Design review of the part built by this model. Coordinates are the model's own, in mm. Face numbers are marked on the shaded views. A direction names the side the tool comes from. Round coordinates to 2 decimals unless told otherwise and drop trailing zeros. Loops run counter-clockwise (first coordinate to the right, second up) from the corner with the lowest first, then second, coordinate; pieces in that order, holes last. Notation, with made-up numbers: (-17.75, 54) - (14.25, 54) arc R20 ccw to (14.25, 84) - close; hole circle Ø10 at (-36, 67). An arc over 180 degrees is marked (long way). Answer as CSV lines item,"result". Start each with the question number.
(1) Wall thickness on L1, parallel to Z at x = 2.75, y = -2; L2, parallel to Y at x = 0, z = 5.5; L3, parallel to Y at x = 0.5, z = 9.5: over which ranges is each line inside the solid? List them lowest first.
(2) Consider section B-B (z = -2). Give the boundary of the cut face in (x, y), and give its area (3 significant figures).
(3) Consider section C-C (x = -2.75). Give the boundary of the cut face in (y, z), and give its area (3 significant figures).
(4) For the marked faces 1 and 2, list the 3-axis set-ups (+Z, -Z, +X, -X, +Y, -Y) from which the entire face can be reached by the end or side of a thin tool; tool diameter is ignored.
(5) Consider section D-D (z = 12). Give the boundary of the cut face in (x, y), and give its area (3 significant figures).
(6) For P1, Ø1, axis at y = 1, z = -16.5, coming from the +X side; P2, Ø1.5, axis at x = 0, y = -3, coming from the +Z side; P3, Ø4, axis at y = -2, z = 5, coming from the -X side, all flat-tipped, find the tip position at first contact; note any pin that passes through.
(7) Consider section A-A (y = 0). Give the boundary of the cut face in (x, z), and give its area (3 significant figures).
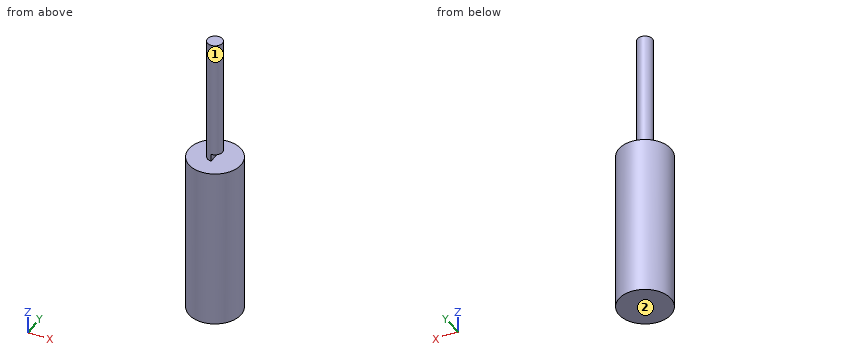
from build123d import *

# Parameters (mm, degrees)
F0_R     = 3.5
F1_DEPTH = 22
F2_START = 1
F2_DEPTH = 16
F3_DEPTH = 1


# Not quite as in the source:
# - a feature names something its author has since deleted; it is built from what else it names


with BuildPart() as f1:
    # F0 (on Top) → F1 (new body)
    with BuildSketch(Plane.XY):
        Circle(F0_R)
        with BuildLine():
            ThreePointArc((0, 1), (0.7071067812, 0.7071067812), (1, 0))
            ThreePointArc((1, 0), (0.7071067812, -0.7071067812), (0, -1))
            ThreePointArc((0, -1), (-1, 0), (0, 1))
        make_face(mode=Mode.SUBTRACT)
        with BuildLine():
            Line((0, 0), (0, 1))
            ThreePointArc((0, 1), (-1, 0), (0, -1))
            Line((0, -1), (0, 0))
        make_face()
        with BuildLine():
            ThreePointArc((0, -1), (0.7071067812, -0.7071067812), (1, 0))
            ThreePointArc((1, 0), (0.7071067812, 0.7071067812), (0, 1))
            Line((0, 1), (0, 0))
            Line((0, 0), (0, -1))
        make_face()
    extrude(amount=-F1_DEPTH)



with BuildPart() as f2:
    # F0 (on Top) → F2 (new body)
    with BuildSketch(Plane.XY.offset(F2_START)):
        with BuildLine():
            Line((0, 0), (0, 1))
            ThreePointArc((0, 1), (-1, 0), (0, -1))
            Line((0, -1), (0, 0))
        make_face()
        with BuildLine():
            ThreePointArc((0, -1), (0.7071067812, -0.7071067812), (1, 0))
            ThreePointArc((1, 0), (0.7071067812, 0.7071067812), (0, 1))
            Line((0, 1), (0, 0))
            Line((0, 0), (0, -1))
        make_face()
    extrude(amount=F2_DEPTH)


with BuildPart() as f1_1:
    add(f1.part)

    add(f2.part)  # F3 merges F2
    # F0 (on Top) → F3 (join)
    with BuildSketch(Plane.XY):
        with BuildLine():
            Line((0, 0), (0, 1))
            ThreePointArc((0, 1), (-1, 0), (0, -1))
            Line((0, -1), (0, 0))
        make_face()
    extrude(amount=F3_DEPTH)


solid = f1_1.part
Determined:
1,L1,"z = -22 to 0"
1,L2,"y = -1 to 1"
1,L3,"y = -0.87 to 0.87"
2,outline,"circle Ø7 at (0, 0)"
2,area,"38.5 mm^2"
3,outline,"(-2.17, -22) - (2.17, -22) - (2.17, 0) - (-2.17, 0) - close"
3,area,"95.3 mm^2"
4,face 1,"+Z"
4,face 2,"-Z, +X, -X, +Y, -Y"
5,outline,"circle Ø2 at (0, 0)"
5,area,"3.14 mm^2"
6,P1,"stops at x = 3.46"
6,P2,"stops at z = 0"
6,P3,"stops at x = -1"
7,outline,"(-3.5, -22) - (3.5, -22) - (3.5, 0) - (0, 0) - (0, 1) - (1, 1) - (1, 17) - (-1, 17) - (-1, 0) - (-3.5, 0) - close"
7,area,"187 mm^2"
